from build123d import *

# Parameters (mm, degrees)
SKICA1_R        = 11.5
SKICA1_R_2      = 10
VYSUNOUT1_DEPTH = 20
ZKOSIT1_SIZE    = 0.5
ZKOSIT1_SIZE2   = 0.288675135
ZKOSIT2_SIZE    = 0.461880215
ZKOSIT2_SIZE2   = 0.8


with BuildPart() as part:
    # Skica1 → Vysunout1 (new body)
    with BuildSketch(Plane.XY):
        Circle(SKICA1_R)
        Circle(SKICA1_R_2, mode=Mode.SUBTRACT)
    extrude(amount=VYSUNOUT1_DEPTH)

    # Zkosit1
    zkosit1_edges = [part.edges().sort_by_distance(p)[0] for p in [
        (-10, 0, 20),
    ]]
    zkosit1_side = [part.faces().sort_by_distance(p)[0] for p in [
        (-10, 0, 10),
    ]]
    chamfer(zkosit1_edges, length=ZKOSIT1_SIZE, length2=ZKOSIT1_SIZE2, reference=zkosit1_side[0])

    # Zkosit2
    zkosit2_edges = [part.edges().sort_by_distance(p)[0] for p in [
        (-11.5, 0, 0),
    ]]
    zkosit2_side = [part.faces().sort_by_distance(p)[0] for p in [
        (-11.174730881, 0, 0),
    ]]
    chamfer(zkosit2_edges, length=ZKOSIT2_SIZE, length2=ZKOSIT2_SIZE2, reference=zkosit2_side[0])


solid = part.part
Read the model definition and answer for the solid it produces. Units are mm, in the model's axes. Give positions to 0.01 mm unless a question says otherwise; leave off trailing zeros. Loops run counter-clockwise (first coordinate to the right, second up) from the corner with the lowest first, then second, coordinate; pieces in that order, holes last. Notation, with made-up numbers: (40, 69) -> (70, 69) arc R19 ccw to (70, 94) -> close; hole circle Ø6 at (29.5, 36.25). An arc over 180 degrees is marked (long way). Use a Markdown table: item, result.
Q1. Determine the mould class of faces 1 (the face through (-1.5, 11.4, 10.3)), 2 (the face through (-2, 10, 0)), 3 (the face through (-2.17, -9.76, 9.61)) for opening direction Y: pulls with the +Y half, pulls with the -Y half, needs draft (parallel to the pull), parting line crosses it, or undercut.
Solved:
| item | result |
|---|---|
| face 1 | parting line crosses it |
| face 2 | needs draft |
| face 3 | undercut |
Q2. Find the intervals of material crossed by line 1 along Y through (x, z) = (0, 8.75); line 2 along X through (y, z) = (-5, 1); line 3 along X through (y, z) = (-5.5, 6), in increasing order.
Solved:
| item | result |
|---|---|
| line 1 | y = -11.5 to -10, 10 to 11.5 |
| line 2 | x = -10.36 to -8.66, 8.66 to 10.36 |
| line 3 | x = -10.1 to -8.35, 8.35 to 10.1 |
Q3. Each of these flat-tipped pins is pushed along its axis until it touches: pin 1 (8 mm diameter, centred on y = 4.5, z = 3.5, fed in from +X); pin 2 (6 mm diameter, centred on y = 6.5, z = 5, fed in from -X); pin 3 (8 mm diameter, centred on x = -5, z = 6, fed in from -Y). Where does it stop, or does it pass through?
Solved:
| item | result |
|---|---|
| pin 1 | stops at x = 11.49 |
| pin 2 | stops at x = -10.95 |
| pin 3 | stops at y = -11.46 |
Q4. Section A-A, the plane x = 0 is taken. Determine the outline of the cut face in (y, z), then the cut area to 3 significant figures.
Solved:
| item | result |
|---|---|
| outline | (-11.5, 0.8) -> (-11.04, 0) -> (-10, 0) -> (-10, 19.5) -> (-10.29, 20) -> (-11.5, 20) -> close; (10, 0) -> (11.04, 0) -> (11.5, 0.8) -> (11.5, 20) -> (10.29, 20) -> (10, 19.5) -> close |
| area | 59.5 mm^2 |
Q5. Section C-C, the plane z = 2.5 is taken. Determine the outline of the cut face in (x, y), then the cut area to 3 significant figures.
Solved:
| item | result |
|---|---|
| outline | circle Ø23 at (0, 0); hole circle Ø20 at (0, 0) |
| area | 101 mm^2 |
